Design review of the part shown in the three views and the two pictorial views. Dimensions are in mm from the part's minimum x, y and z. A direction names the side the tool comes from. Coordinates: 2 decimals unless noted, no trailing zeros. Loops run counter-clockwise (first coordinate to the right, second up) from the corner with the lowest first, then second, coordinate; pieces in that order, holes last. Notation, with made-up numbers: (29, 52.25) -> (65, 52.25) arc R26 cw to (65, 78.25) -> close; hole circle Ø3 at (46.5, 61.5). An arc over 180 degrees is marked (long way). One line per item, written item: value.
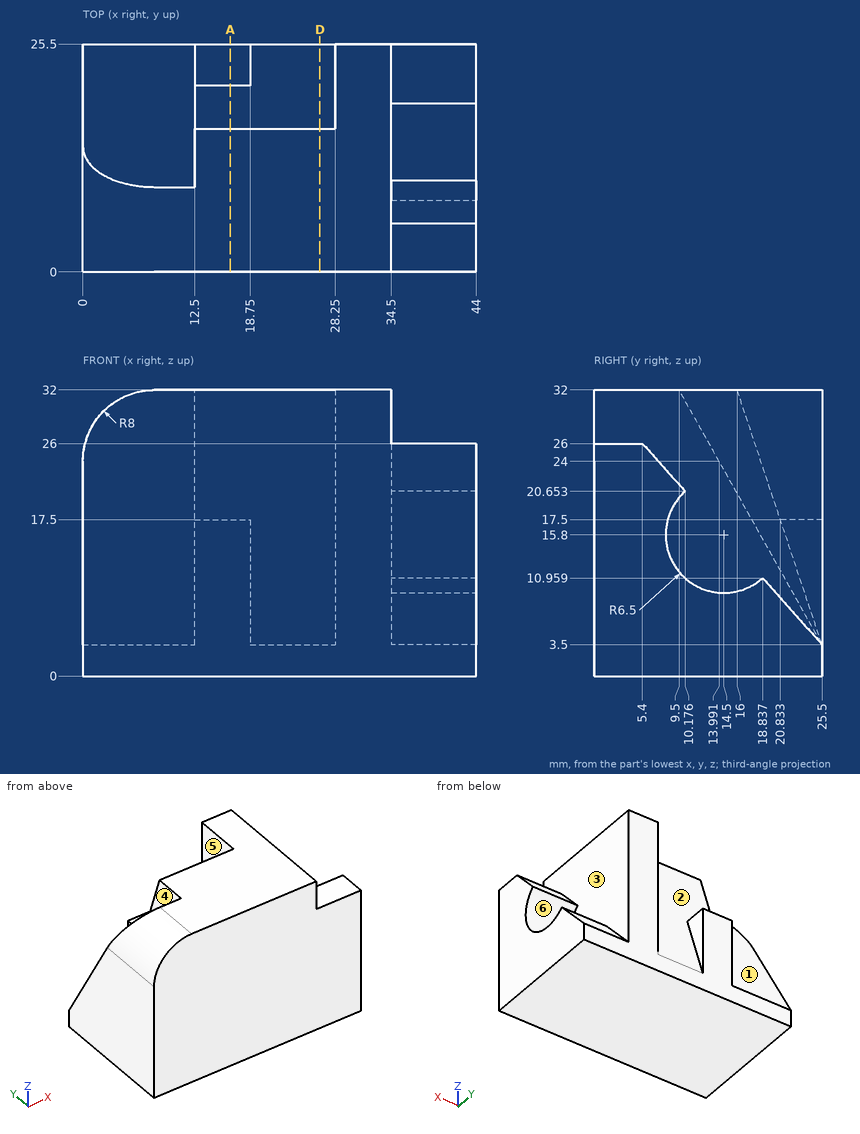
1. Take a section at A-A, the plane x = 16.5. Give the boundary of the cut face in (y, z).
Return value:
outline: (0, 0) -> (25.5, 0) -> (25.5, 17.5) -> (20.83, 17.5) -> (16, 32) -> (0, 32) -> close
2. Take a section at D-D, the plane x = 26.5. Give the boundary of the cut face in (y, z).
Return value:
outline: (0, 0) -> (25.5, 0) -> (25.5, 3.5) -> (16, 32) -> (0, 32) -> close
3. The part is to be moulded in two halves that separate along X. For the marked faces 1, 2 and 3, say which applies: pulls with the +X half, pulls with the -X half, needs draft (parallel to the pull), parting line crosses it, or undercut.
Return value:
face 1: needs draft
face 2: undercut
face 3: pulls with the +X half
4. To check wall thickness, follow probe 1 along Y at (x, z) = (19, 8); probe 2 along Z at (x, y) = (35, 4.75); probe 3 along X at (y, z) = (22.25, 8.5). State the ranges of each line that lie inside material, in increasing order. Write a range as from..to.
Return value:
probe 1: y = 0..24
probe 2: z = 0..26
probe 3: x = 0..34.5
5. Insertion check: pin 1 Ø1.4 at (x, y) = (17, 24) entering from +Z; pin 2 Ø3.5 at (y, z) = (22, 11.5) entering from +X; pin 3 Ø2.5 at (x, y) = (41.5, 3.5) entering from +Z. Each pin has a flat end and moves straight along its axis. Give the tip position at first contact, or say it passes through.
Return value:
pin 1: stops at z = 17.5
pin 2: stops at x = 34.5
pin 3: stops at z = 26
6. For the marked faces 4, 5 and 6, list the 3-axis set-ups (+Z, -Z, +X, -X, +Y, -Y) from which the entire face can be reached by the end or side of a thin tool; tool diameter is ignored.
Return value:
face 4: +Z, -X, +Y
face 5: +Z, +Y
face 6: +X
